Part print with two shaded views. Sizes in mm from the minimum x, y, z corner. A direction names the side the tool comes from. Give positions to 0.01 mm unless a question says otherwise; leave off trailing zeros. Write each loop counter-clockwise with the first axis right and the second up, starting at its lowest first coordinate (ties: lowest second). Pieces come first, ordered by that corner, then holes.
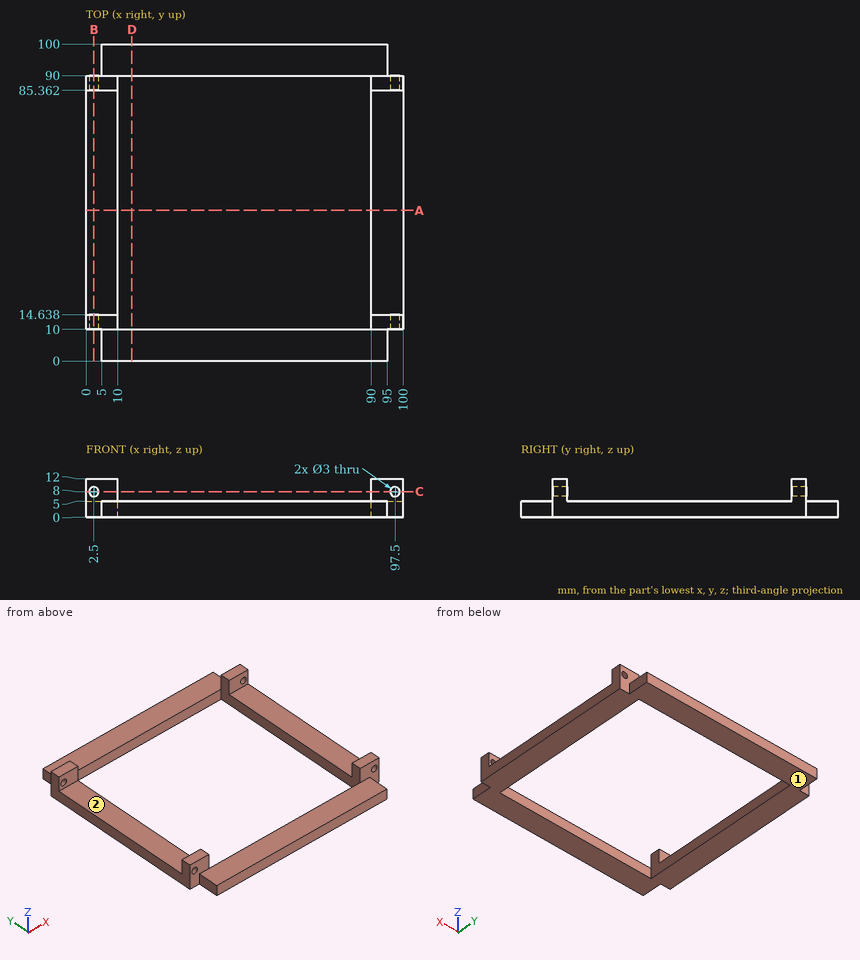
1) Drill centre lines: L1, parallel to Y at x = 21, z = 1.25; L2, parallel to Z at x = 97.5, y = 89.05. Where is each one in solid material? Low to high.
Check result:
L1: y = 0 to 10, 90 to 100
L2: z = 0 to 6.5, 9.5 to 12
2) Flat gauge pins, fed straight in: P1, Ø6, axis at x = 25, z = 5, coming from the -Y side; P2, Ø5, axis at x = 2.5, z = 8, coming from the -Y side; P3, Ø5, axis at x = 40.5, y = 3.5, coming from the +Z side; P4, Ø4, axis at y = 7.5, z = 2.5, coming from the +X side. Where does each tip first touch, or does it go through?
Check result:
P1: stops at y = 0
P2: stops at y = 10
P3: stops at z = 5
P4: stops at x = 95
3) Saw through at A-A (y = 47.5). Write the cut outline in (x, z).
Check result:
outline: (0, 0) - (10, 0) - (10, 5) - (0, 5) - close; (90, 0) - (100, 0) - (100, 5) - (90, 5) - close
4) Saw through at B-B (x = 2.5). Write the cut outline in (y, z).
Check result:
outline: (10, 0) - (90, 0) - (90, 6.5) - (85.36, 6.5) - (85.36, 5) - (14.64, 5) - (14.64, 6.5) - (10, 6.5) - close; (10, 9.5) - (14.64, 9.5) - (14.64, 12) - (10, 12) - close; (85.36, 9.5) - (90, 9.5) - (90, 12) - (85.36, 12) - close
5) 3-axis set-ups, long thin cutter, end or side, ignore diameter. For the marked faces 1 and 2: which of +Z, -Z, +X, -X, +Y, -Y reach the whole face in a straight line?
Check result:
face 1: -Z, +X, -X, +Y, -Y
face 2: +Z, +X, -X
6) Saw through at C-C (z = 8). State how many separate pieces and enclosed holes the cut face has, and give its area (3 significant figures).
Check result:
separate pieces: 8
enclosed holes: 0
area: 130 mm2
